Could you check a few things on this drawing? It's one solid part, dimensions in mm from its lowest x, y, z. A direction names the side the tool comes from. Round coordinates to 2 decimals unless told otherwise and drop trailing zeros. Loops run counter-clockwise (first coordinate to the right, second up) from the corner with the lowest first, then second, coordinate; pieces in that order, holes last. Notation, with made-up numbers: M 86,81.25 L 93,81.25 A15 cw 93,105.25 Z; hole C 25.5,66 d10. An arc over 180 degrees is marked long. Answer as a JSON object with one key per item and string values.
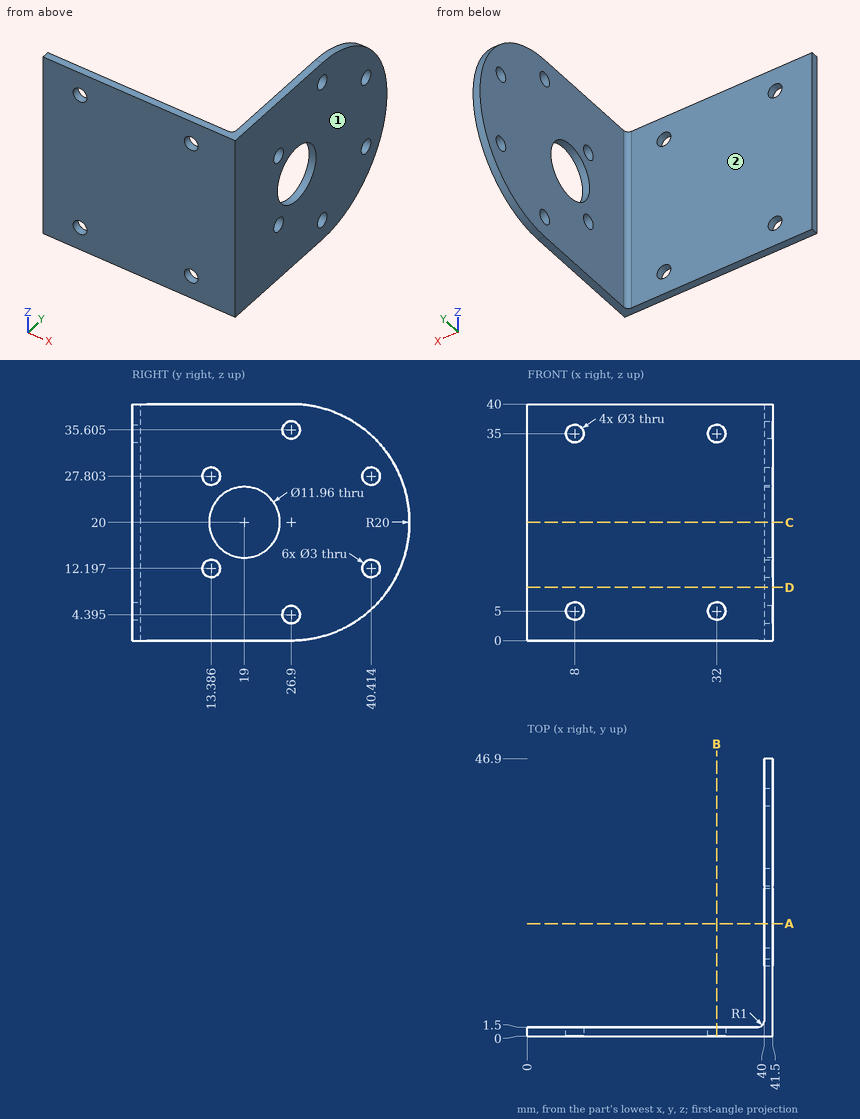
Item 1: I want a section at A-A, the plane y = 19. Please give me the cut outline in (x, z).
Resolved:
{"outline": "M 40,0 L 41.5,0 L 41.5,14.02 L 40,14.02 Z; M 40,25.98 L 41.5,25.98 L 41.5,40 L 40,40 Z"}
Item 2: Please list where these lines run through material, in increasing order: probe 1 along Z at (x, y) = (8, 0.8); probe 2 along Z at (x, y) = (40.6, 26.9) (1 decimal); probe 3 along Y at (x, z) = (4, 25). Write a range as from..to.
Resolved:
{"probe 1": "0..3.5, 6.5..33.5, 36.5..40", "probe 2": "0..2.9, 5.9..34.1, 37.1..40", "probe 3": "0..1.5"}
Item 3: I want a section at C-C, the plane z = 20. Please give me the cut outline in (x, y).
Resolved:
{"outline": "M 0,0 L 41.5,0 L 41.5,13.02 L 40,13.02 L 40,2.5 A1 cw 39,1.5 L 0,1.5 Z; M 40,24.98 L 41.5,24.98 L 41.5,46.9 L 40,46.9 Z"}
Item 4: I want a section at D-D, the plane z = 9. Please give me the cut outline in (x, y).
Resolved:
{"outline": "M 0,0 L 41.5,0 L 41.5,43.6 L 40,43.6 L 40,2.5 A1 cw 39,1.5 L 0,1.5 Z"}
Item 5: I'm going to push flat-ended pins straight in: pin 1 Ø4 at (y, z) = (26.9, 4.395) entering from -X; pin 2 Ø1.5 at (x, z) = (6.5, 24.5) entering from +Y. Where does each tip first touch, or does it pass through?
Resolved:
{"pin 1": "x = 40", "pin 2": "y = 1.5"}
Item 6: On a 3-axis mill with a long thin cutter (end or side, diameter ignored), from which of +Z, -Z, +X, -X, +Y, -Y can I reach the whole of each face in a straight line? I mean the marked faces 1 and 2. Say none if no direction works.
Resolved:
{"face 1": "+Z, -Z, +X, +Y, -Y", "face 2": "+Z, -Z, -X, +Y"}
Item 7: I want a section at B-B, the plane x = 32. Please give me the cut outline in (y, z).
Resolved:
{"outline": "M 0,0 L 1.5,0 L 1.5,3.5 L 0,3.5 Z; M 0,6.5 L 1.5,6.5 L 1.5,33.5 L 0,33.5 Z; M 0,36.5 L 1.5,36.5 L 1.5,40 L 0,40 Z"}
